Build history of the part. All positions in model axes, mm. Face numbers are marked on the shaded views. A direction names the side the tool comes from. Give positions to 0.01 mm unless a question says otherwise; leave off trailing zeros. Order: outer loops, then holes, each group sorted by start corner. A loop starts at its lowest first (then second) coordinate and runs counter-clockwise, first axis right, second up. Notation, with made-up numbers: (-0.75, 85.25) - (47.25, 85.25) arc R10 cw to (47.25, 103.25) - close; hole circle Ø7 at (39.5, -38). An arc over 180 degrees is marked (long way). Use a Markdown table: item, result. Add a question column.
(1) Flat gauge pins, fed straight in: pin 1 (3 mm diameter, centred on x = 12.5, y = -3, fed in from -Z); pin 2 (3 mm diameter, centred on x = -25.5, y = 4, fed in from -Z); pin 3 (3 mm diameter, centred on x = -7.5, y = 2, fed in from -Z). Where does each tip first touch, or does it go through?
(2) Slice it at C-C (z = -7.75). Write the cut outline in (x, y).
(3) Slice it at B-B (y = 0.25). Write the cut outline in (x, z), then the cut area to 3 significant figures.
(4) Slice it at A-A (x = 37.5). Write the cut outline in (y, z), then the cut area to 3 significant figures.
(5) Which spindle directions (+Z, -Z, +X, -X, +Y, -Y) get a long thin tool onto all of the face, cutting with end or side? Do the marked faces 1 and 2. Say none if no direction does.
(6) Wall check: line 1 (Z direction, x = 36.5, y = 2); line 2 (Y direction, x = -5, z = -3.75); line 3 (Y direction, x = -37.5, z = 0.6). Give the ranges that are in metal, low to high.
(7) Slice it at D-D (z = -1). Write the cut outline in (x, y), then the cut area to 3 significant figures.
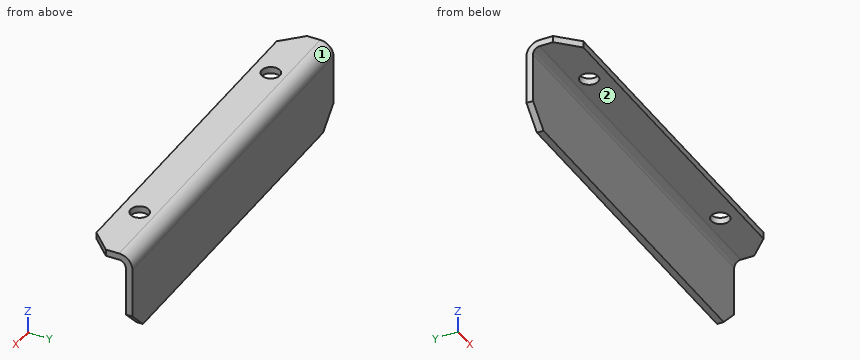
Autodesk Inventor part; units mm, degrees
ref_plane "YZ Plane" through (0, 0, 0) normal (1, 0, 0) x (0, 1, 0)
ref_plane "XZ Plane" through (0, 0, 0) normal (0, 1, 0) x (-1, 0, 0)
ref_plane "XY Plane" through (0, 0, 0) normal (0, 0, 1) x (1, 0, 0)
sketch "Sketch1" plane through (0, 0, 0) normal (0, 0, 1) x (1, 0, 0)
  line L0 (-57.5, -7) -> (57.5, -7)
  line L1 (57.5, -7) -> (57.5, 7)
  line L2 (57.5, 7) -> (-57.5, 7)
  line L3 (-57.5, 7) -> (-57.5, -7)
  line L4 (-57.5, -7) -> (57.5, 7) construction
  line L5 (57.5, -7) -> (-57.5, 7) construction
  point P0 (0, 0)
  dimension "d0" = 115
  dimension "d1" = 14
extrude "Plate1" add sketch "Sketch1" along normal blind 2
sketch "Sketch2" plane through (57.5, 5, 2) normal (0, 1, 0) x (-1, 0, 0)
  line L0 (115, 0) -> (0, 0)
  line L1 (0, 0) -> (0, -25)
  line L2 (0, -25) -> (115, -25)
  line L3 (115, -25) -> (115, 0)
edge flange "Flange1" height 25 angle 90 thickness 2 bend radius 2 thickness toward (0, 1, 0) relief tear relief width 2 relief depth 1 edges at (0, 7, 0) wall of the first edge with corners at (-57.5, 5, 2) (57.5, 5, 2) (57.5, 5, -23) (-57.5, 5, -23)
bend "Bend1"
corner "Corner1"
chamfer "Corner Chamfer1" distance 6 angle 45 4 edges at (-57.5, -7, 1) (57.5, -7, 1) (-57.5, 6, -23) (57.5, 6, -23)
sketch "Sketch3" plane through (0, 0, 2) normal (0, 0, 1) x (1, 0, 0)
  circle A0 centre (-37.5, -132.5) radius 2.9585
  circle A1 centre (37.5, -132.5) radius 2.9585
  circle A2 centre (-5, -1.3494) radius 3.1
  point P0 (0, 0)
  point P1 (-37.5, -1.3494)
  point P2 (37.5, -1.3494)
hole "Hole1" at (-37.5, -1.3494, 2) at (37.5, -1.3494, 2) direction (0, 0, -1) diameter 5.5 depth 2 tip angle 118
sketch "Sketch4" plane through (0, 0, 0) normal (0, 0, -1) x (-1, 0, 0)
  point P0 (0, 0)
equation "\"d21\" = Thickness"
equation "\"d3\" = BendReliefWidth"
equation "\"d4\" = BendReliefDepth"
equation "\"d5\" = MinimumRemnant"
equation "\"d6\" = BendRadius"
equation "\"d9\" = BendRadius"
equation "\"d10\" = CornerReliefSize"
equation "\"d11\" = GapSize"
equation "\"d12\" = JacobiRadiusSize"
equation "\"BendRadius\" = Thickness"
equation "\"BendReliefWidth\" = Thickness"
equation "\"BendReliefDepth\" = 0.5 * Thickness"
equation "\"CornerReliefSize\" = 4 * Thickness"
equation "\"MinimumRemnant\" = 2 * Thickness"
equation "\"TransitionRadius\" = BendRadius"
equation "\"JacobiRadiusSize\" = BendRadius"
equation "\"GapSize\" = Thickness"
equation "\"d2\" = BendRadius"
Solution:
| question | item | result |
|---|---|---|
| 1 | pin 1 | z = 0 |
| 1 | pin 2 | z = -23 |
| 1 | pin 3 | z = -0.06 |
| 2 | outline | (-57.5, 5) - (57.5, 5) - (57.5, 7) - (-57.5, 7) - close |
| 3 | outline | (-57.5, 0) - (-39.74, 0) - (-39.74, 2) - (-57.5, 2) - close; (-35.26, 0) - (35.26, 0) - (35.26, 2) - (-35.26, 2) - close; (39.74, 0) - (57.5, 0) - (57.5, 2) - (39.74, 2) - close |
| 3 | area | 212 mm2 |
| 4 | outline | (-7, 0) - (-4.1, 0) - (-4.1, 2) - (-7, 2) - close; (1.4, 0) - (3, 0) arc R2 cw to (5, -2) - (5, -23) - (7, -23) - (7, -2) arc R4 ccw to (3, 2) - (1.4, 2) - close |
| 4 | area | 60.4 mm2 |
| 5 | face 1 | +Z, +X, -X, +Y |
| 5 | face 2 | -Z, +X, -X, -Y |
| 6 | line 1 | 0 to 2 |
| 6 | line 2 | 5 to 7 |
| 6 | line 3 | -7 to -4.1, 1.4 to 6.04 |
| 7 | outline | (-57.5, 4.73) - (57.5, 4.73) - (57.5, 6.87) - (-57.5, 6.87) - close |
| 7 | area | 246 mm2 |
